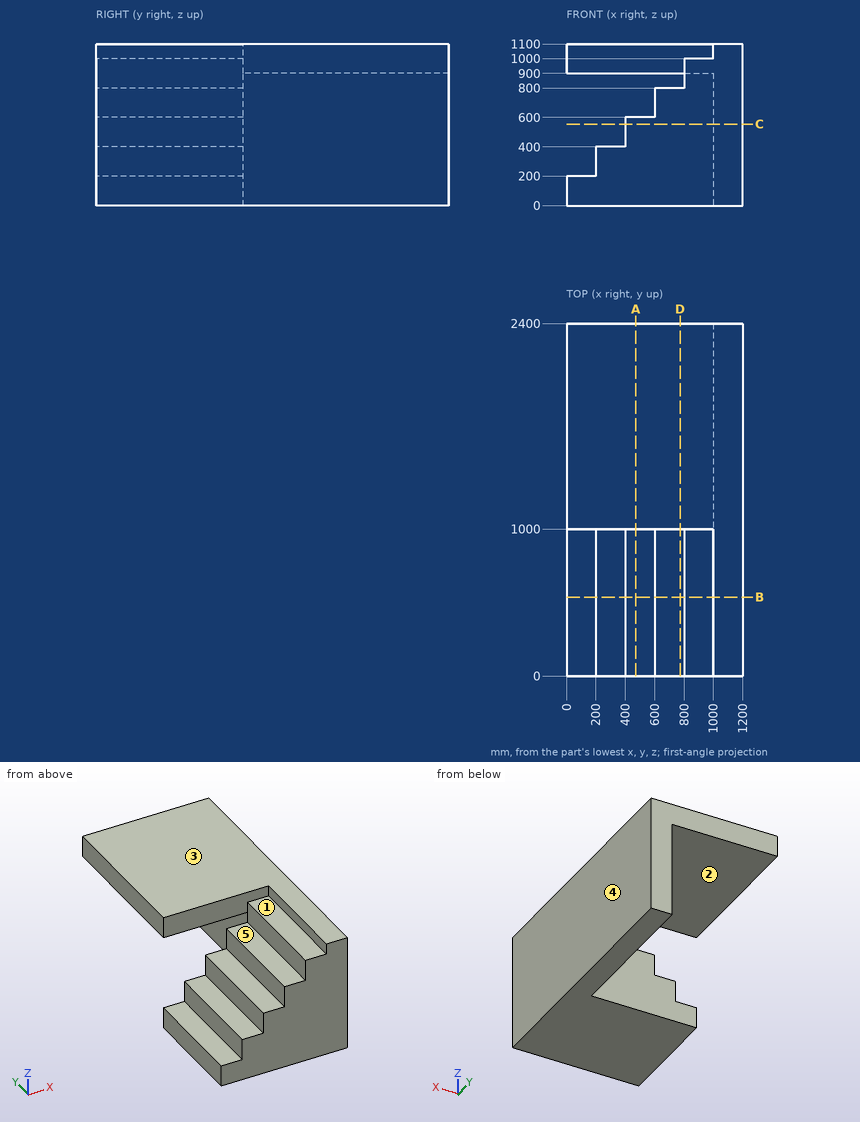
For this review, use the dimensioned drawing (mm, ordinates from the lowest corner) and the shaded views. A direction names the side the tool comes from. Give positions to 0.01 mm unless a question says otherwise; leave off trailing zeros. Loops run counter-clockwise (first coordinate to the right, second up) from the corner with the lowest first, then second, coordinate; pieces in that order, holes last. Notation, with made-up numbers: (42.25, -21.5) -> (54.25, -21.5) arc R14 ccw to (54.25, -4.5) -> close; hole circle Ø11 at (10, 82.5). An arc over 180 degrees is marked (long way). One line per question, with ' | ' between items. Start each with the question number.
(1) We need section D-D (x = 772.5). State the section outline as (y, z) points.
(2) For line 1 (Z direction, x = 907.5, y = 493); line 2 (Z direction, x = 613.5, y = 735.5); line 3 (Y direction, x = 511.5, z = 952), list the stretches that pass through material, from the lowest coordinate up.
(3) We need section A-A (x = 471). State the section outline as (y, z) points, and give its area (3 significant figures).
(4) We need section C-C (z = 554). State the section outline as (x, y) points.
(5) For the marked faces 1, 2, 3, 4 and 5, list the 3-axis set-ups (+Z, -Z, +X, -X, +Y, -Y) from which the entire face can be reached by the end or side of a thin tool; tool diameter is ignored.
(6) Insertion check: P1, Ø4, axis at y = 2111.5, z = 420, coming from the -X side. The pin has a flat end and moves straight along its axis. Give the tip position at first contact, or say it passes through.
(7) We need section B-B (y = 536.5). State the section outline as (x, z) points.
The answers:
1) outline: (0, 0) -> (1000, 0) -> (1000, 800) -> (0, 800) -> close; (1000, 900) -> (2400, 900) -> (2400, 1100) -> (1000, 1100) -> close
2) line 1: z = 0 to 1000 | line 2: z = 0 to 800 | line 3: y = 1000 to 2400
3) outline: (0, 0) -> (1000, 0) -> (1000, 600) -> (0, 600) -> close; (1000, 900) -> (2400, 900) -> (2400, 1100) -> (1000, 1100) -> close | area: 880,000 mm^2
4) outline: (400, 0) -> (1200, 0) -> (1200, 2400) -> (1000, 2400) -> (1000, 1000) -> (400, 1000) -> close
5) face 1: +Z, -X, -Y | face 2: -Z, -X, +Y | face 3: +Z, +X, -X, +Y, -Y | face 4: +Z, -Z, +X, +Y, -Y | face 5: +Z, -X, +Y, -Y
6) P1: stops at x = 1000
7) outline: (0, 0) -> (1200, 0) -> (1200, 1100) -> (1000, 1100) -> (1000, 1000) -> (800, 1000) -> (800, 800) -> (600, 800) -> (600, 600) -> (400, 600) -> (400, 400) -> (200, 400) -> (200, 200) -> (0, 200) -> close
